Geometry: final body of the model. Coordinates: model frame, mm. Face numbers are marked on the shaded views. A direction names the side the tool comes from. Coordinates: 2 decimals unless noted, no trailing zeros. Loops run counter-clockwise (first coordinate to the right, second up) from the corner with the lowest first, then second, coordinate; pieces in that order, holes last. Notation, with made-up numbers: (21.5, -36.75) - (50.5, -36.75) arc R16 ccw to (50.5, -11.75) - close; hole circle Ø10 at (6, 86). An arc over 180 degrees is marked (long way). Return JSON: item names as keys, results as strings.
from build123d import *

# Parameters (mm, degrees)
SKETCH1_W                    = 35
SKETCH1_H                    = 25
BASE_FLANGE1_DEPTH           = 0.7
EDGE_FLANGE1_STRIP_W         = 3.8
EDGE_FLANGE1_STRIP_H         = 0.7
EDGE_FLANGE1_STRIP_CUT_DEPTH = 25
EDGE_FLANGE1_DEPTH           = 25
SKETCH10_R                   = 1.6
CUT_EXTRUDE1_DEPTH           = 0.7


# Sheet-metal steps are written as plain solids
with BuildPart() as part:
    # Sketch1 → Base-Flange1 (new body)
    with BuildSketch(Plane.XY):
        Rectangle(SKETCH1_W, SKETCH1_H)
    extrude(amount=-BASE_FLANGE1_DEPTH)

    # Edge-Flange1 strip (across the edge) → Edge-Flange1 strip cut (cut)
    with BuildSketch(Plane(origin=(17.5, 12.5, -0.7), x_dir=(-1, 0, 0), z_dir=(0, -1, 0))):
        with Locations((-1.4, -0.35)):
            Rectangle(EDGE_FLANGE1_STRIP_W, EDGE_FLANGE1_STRIP_H)
    extrude(amount=EDGE_FLANGE1_STRIP_CUT_DEPTH, mode=Mode.SUBTRACT)

    # Edge-Flange1 section (across the edge) → Edge-Flange1 (add)
    with BuildSketch(Plane(origin=(17.5, 12.5, -0.7), x_dir=(-1, 0, 0), z_dir=(0, -1, 0))):
        with BuildLine():
            Line((-0.7, 0.5), (-0.7, 15))
            Line((-0.7, 15), (0, 15))
            Line((0, 15), (0, 0.5))
            ThreePointArc((0, 0.5), (0.146446609, 0.146446609), (0.5, 0))
            Line((0.5, 0), (0.5, -0.7))
            ThreePointArc((0.5, -0.7), (-0.348528137, -0.348528137), (-0.7, 0.5))
        make_face()
    extrude(amount=EDGE_FLANGE1_DEPTH)

    # Sketch10 → Cut-Extrude1 (cut)
    with BuildSketch(Plane.ZY.offset(-17.5)):
        with Locations((-10.7, 2.5)):
            Circle(SKETCH10_R)
    extrude(amount=-CUT_EXTRUDE1_DEPTH, mode=Mode.SUBTRACT)


solid = part.part
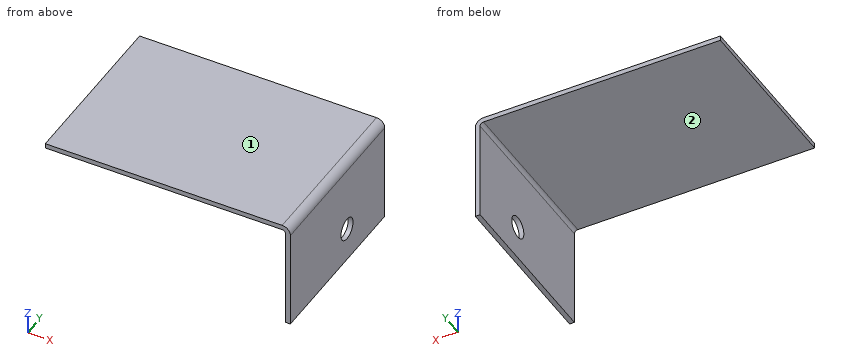
Item 1: First-contact query: pin 1 Ø1 at (x, z) = (12.5, -2) entering from -Y (3 decimals); pin 2 Ø3 at (y, z) = (-4, -4.5) entering from -X; pin 3 Ø12.5 at (x, y) = (7, 2) entering from -Z. Flat tips, straight axial feed; report the tip coordinate or a pass-through.
Worked out:
{"pin 1": "through", "pin 2": "x = 17.5", "pin 3": "z = -0.7"}
Item 2: Section query D-D, the plane x = -7.5. Return loops of the section in (y, z), and give its area (3 significant figures).
Worked out:
{"outline": "(-12.5, -0.7) - (12.5, -0.7) - (12.5, 0) - (-12.5, 0) - close", "area": "17.5 mm^2"}
Item 3: Section query A-A, the plane z = -10.7. Return loops of the section in (x, y).
Worked out:
{"outline": "(17.5, -12.5) - (18.2, -12.5) - (18.2, 0.9) - (17.5, 0.9) - close; (17.5, 4.1) - (18.2, 4.1) - (18.2, 12.5) - (17.5, 12.5) - close"}
Item 4: Ray query, probe 1 along Y at (x, z) = (17.75, -10.7); probe 2 along X at (y, z) = (5.5, -13.5); probe 3 along Z at (x, y) = (2.5, 4). Return the intervals inside material, ascending. Write a range as from..to.
Worked out:
{"probe 1": "-12.5..0.9, 4.1..12.5", "probe 2": "17.5..18.2", "probe 3": "-0.7..0"}
Item 5: Section query C-C, the plane y = 7. Return loops of the section in (x, z), and give its area (3 significant figures).
Worked out:
{"outline": "(-17.5, -0.7) - (17, -0.7) arc R0.5 cw to (17.5, -1.2) - (17.5, -15.7) - (18.2, -15.7) - (18.2, -1.2) arc R1.2 ccw to (17, 0) - (-17.5, 0) - close", "area": "35.2 mm^2"}
Item 6: Reachability of the marked faces 1 and 2 from +Z, -Z, +X, -X, +Y, -Y: full face, straight path, thin tool, end or side. Return the list, or none.
Worked out:
{"face 1": "+Z, +X, -X, +Y, -Y", "face 2": "-Z, -X, +Y, -Y"}
Item 7: Section query B-B, the plane y = 2.5. Return loops of the section in (x, z).
Worked out:
{"outline": "(-17.5, -0.7) - (17, -0.7) arc R0.5 cw to (17.5, -1.2) - (17.5, -9.1) - (18.2, -9.1) - (18.2, -1.2) arc R1.2 ccw to (17, 0) - (-17.5, 0) - close; (17.5, -15.7) - (18.2, -15.7) - (18.2, -12.3) - (17.5, -12.3) - close"}
